Could you check a few things on this model? Use its own coordinates, in mm. A direction names the side the tool comes from. Give positions to 0.01 mm unless a question says otherwise; leave off trailing zeros. Write each loop counter-clockwise with the first axis right and the second up, starting at its lowest first coordinate (ties: lowest second). Pieces come first, ordered by that corner, then holes. Notation, with made-up numbers: M -32.5,82.5 L -25.5,82.5 A27 cw -25.5,102.5 Z; hole C 30,60.5 d5. An arc over 180 degrees is marked long. Answer as CSV lines item,"result". Start each with the question number.
from build123d import *

# Parameters (mm, degrees)
SKETCH_1_W          = 120
SKETCH_1_H          = 155
SKETCH_1_R          = 1.45
SKETCH_1_R_2        = 30.5
SKETCH_1_R_3        = 1.725
SKETCH_1_W_2        = 35
SKETCH_1_H_2        = 28
SKETCH_1_W_3        = 54.975
SKETCH_1_H_3        = 45
SKETCH_1_W_4        = 4.95
SKETCH_1_H_4        = 20
EXTRUDE_1_DEPTH     = 3
FILLET_1_R          = 6
FILLET_2_R          = 10
SKETCH_2_W          = 31.025
SKETCH_2_H          = 25
CUT_EXTRUDE_1_DEPTH = 197.04591299
FILLET_3_R          = 6
FILLET_4_R          = 5
SKETCH_3_R          = 1.5
CUT_EXTRUDE_2_DEPTH = 197.04591299


with BuildPart() as part:
    # 草图1 → 凸台-拉伸1 (new body)
    # profile 1 of 2: a face of its own
    with BuildSketch(Plane.XY):
        with Locations((-60, 77.5)):
            Rectangle(SKETCH_1_W, SKETCH_1_H)
        with Locations((-15, 7.5)):
            Circle(SKETCH_1_R, mode=Mode.SUBTRACT)
        with Locations((-55, 7.5)):
            Circle(SKETCH_1_R, mode=Mode.SUBTRACT)
        with Locations((-15, 147.5)):
            Circle(SKETCH_1_R, mode=Mode.SUBTRACT)
        with Locations((-55, 147.5)):
            Circle(SKETCH_1_R, mode=Mode.SUBTRACT)
        with Locations((-56.5, 92)):
            Circle(SKETCH_1_R_2, mode=Mode.SUBTRACT)
        with Locations((-56.5, 134.5)):
            Circle(SKETCH_1_R_3, mode=Mode.SUBTRACT)
        with Locations((-56.5, 49.5)):
            Circle(SKETCH_1_R_3, mode=Mode.SUBTRACT)
        with Locations((-87.966251763, 123.466251763)):
            Circle(SKETCH_1_R_3, mode=Mode.SUBTRACT)
        with Locations((-87.966251763, 60.533748237)):
            Circle(SKETCH_1_R_3, mode=Mode.SUBTRACT)
        with Locations((-25.033748237, 60.533748237)):
            Circle(SKETCH_1_R_3, mode=Mode.SUBTRACT)
        with Locations((-25.033748237, 123.466251763)):
            Circle(SKETCH_1_R_3, mode=Mode.SUBTRACT)
        with Locations((-12, 92)):
            Circle(SKETCH_1_R_3, mode=Mode.SUBTRACT)
        with Locations((-101, 92)):
            Circle(SKETCH_1_R_3, mode=Mode.SUBTRACT)
        with Locations((-95, 7.5)):
            Circle(SKETCH_1_R, mode=Mode.SUBTRACT)
        with Locations((-95, 147.5)):
            Circle(SKETCH_1_R, mode=Mode.SUBTRACT)
        Polygon((-110, 65), (-110, 15), (-85, 15), (-85, 45), align=None, mode=Mode.SUBTRACT)
        with Locations((-57.5, 29)):
            Rectangle(SKETCH_1_W_2, SKETCH_1_H_2, mode=Mode.SUBTRACT)
        Polygon((-10, 60), (-10, 15), (-30, 15), (-30, 45), align=None, mode=Mode.SUBTRACT)
    # profile 2 of 2: a face of its own
    with BuildSketch(Plane.XY):
        with Locations((27.4875, 105)):
            Rectangle(SKETCH_1_W_3, SKETCH_1_H_3)
        with Locations((41, 102.5)):
            Circle(SKETCH_1_R, mode=Mode.SUBTRACT)
        with Locations((41, 112.5)):
            Circle(SKETCH_1_R, mode=Mode.SUBTRACT)
        with Locations((47.5, 107.5)):
            Rectangle(SKETCH_1_W_4, SKETCH_1_H_4, mode=Mode.SUBTRACT)
    extrude(amount=EXTRUDE_1_DEPTH)

    # 圆角1
    fillet_1_edges = [part.edges().sort_by_distance(p)[0] for p in [
        (-75, 43, 1.5),
        (-75, 15, 1.5),
        (-40, 15, 1.5),
        (-40, 43, 1.5),
        (-110, 65, 1.5),
        (-110, 15, 1.5),
        (-85, 15, 1.5),
        (-85, 45, 1.5),
        (-30, 15, 1.5),
        (-10, 15, 1.5),
        (-10, 60, 1.5),
        (-30, 45, 1.5),
    ]]
    fillet(fillet_1_edges, radius=FILLET_1_R)

    # 圆角2
    fillet_2_edges = [part.edges().sort_by_distance(p)[0] for p in [
        (0, 82.5, 1.5),
        (0, 127.5, 1.5),
    ]]
    fillet(fillet_2_edges, radius=FILLET_2_R)

    # 草图2 → 切除-拉伸1 (cut, through all)
    with BuildSketch(Plane.XY.offset(3)):
        with Locations((17.5125, 105)):
            Rectangle(SKETCH_2_W, SKETCH_2_H)
    extrude(amount=-CUT_EXTRUDE_1_DEPTH, mode=Mode.SUBTRACT)

    # 圆角3
    fillet_3_edges = [part.edges().sort_by_distance(p)[0] for p in [
        (2, 92.5, 1.5),
        (2, 117.5, 1.5),
        (33.025, 117.5, 1.5),
        (33.025, 92.5, 1.5),
    ]]
    fillet(fillet_3_edges, radius=FILLET_3_R)

    # 圆角4
    fillet_4_edges = [part.edges().sort_by_distance(p)[0] for p in [
        (54.975, 82.5, 1.5),
        (0, 0, 1.5),
        (-120, 0, 1.5),
        (-120, 155, 1.5),
        (0, 155, 1.5),
        (54.975, 127.5, 1.5),
    ]]
    fillet(fillet_4_edges, radius=FILLET_4_R)

    # 草图3 → 切除-拉伸2 (cut, through all)
    with BuildSketch(Plane.XY.offset(3)):
        with Locations((45.025, 117.5)):
            Circle(SKETCH_3_R)
        with Locations((49.975, 117.5)):
            Circle(SKETCH_3_R)
        with Locations((45.025, 97.5)):
            Circle(SKETCH_3_R)
        with Locations((49.975, 97.5)):
            Circle(SKETCH_3_R)
    extrude(amount=-CUT_EXTRUDE_2_DEPTH, mode=Mode.SUBTRACT)


solid = part.part
1. Please list where these lines run through material, in increasing order: line 1 (Y direction, x = -56.5, z = 1.2) (3 decimals); line 2 (X direction, y = 59.5, z = 1.2); line 3 (Y direction, x = -104.5, z = 1.1).
2. Imagine slicing it at D-D, the plane y = 141. Please give me the cut outline in (x, z), plus the area to 3 significant figures.
3. Imagine slicing it at B-B, the plane y = 65. Please give me the cut outline in (x, z), plus the area to 3 significant figures.
4. Imagine slicing it at C-C, the plane z = 1.4. State how many separate pieces and enclosed holes the cut face has, plus the area to 3 significant figures.
5. Will these pins go through, and if not, where does the flat tip stop? P1, Ø0.9, axis at y = 26.5, z = 1, coming from the +X side; P2, Ø0.9, axis at x = 21, z = 2, coming from the +Y side; P3, Ø1.5, axis at x = 20.5, z = 1.5, coming from the -Y side.
6. On a 3-axis mill with a long thin cutter (end or side, diameter ignored), from which of +Z, -Z, +X, -X, +Y, -Y can I reach the whole of each face in a straight line? I mean faces 4 (the cylindrical face through (-1, 2, 2)), 5 (the cylindrical face through (-108.289, 16.804, 1.521)). Say none if no direction works.
7. Thinking about a two-plate mould opening in Y: for faces 1 (the cylindrical face through (-119, 153, 2)), 2 (the cylindrical face through (2.85, 79.49, 1.52)), 3 (the cylindrical face through (-80.704, 73.441, 1.479)), which applies, pulls with the +Y half, pulls with the -Y half, needs draft (parallel to the pull), parting line crosses it, or undercut?
8. Imagine slicing it at A-A, the plane x = -37. Please give me the cut outline in (y, z), plus the area to 3 significant figures.
Solutions:
1,line 1,"0 to 15, 43 to 47.775, 51.225 to 61.5, 122.5 to 132.775, 136.225 to 155"
1,line 2,"-120 to -89.35, -86.59 to -26.41, -23.65 to 0"
1,line 3,"0 to 15.02, 58.5 to 155"
2,outline,"M -120,0 L 0,0 L 0,3 L -120,3 Z"
2,area,"360 mm²"
3,outline,"M -120,0 L -70.69,0 L -70.69,3 L -120,3 Z; M -42.31,0 L 0,0 L 0,3 L -42.31,3 Z"
3,area,"275 mm²"
4,separate pieces,"1"
4,enclosed holes,"22"
4,area,"14,600 mm²"
5,P1,"x = 0"
5,P2,"y = 127.5"
5,P3,"y = 82.5"
6,face 4,"+Z, -Z, +X, -Y"
6,face 5,"+Z, -Z"
7,face 1,"pulls with the +Y half"
7,face 2,"pulls with the -Y half"
7,face 3,"undercut"
8,outline,"M 0,0 L 68.55,0 L 68.55,3 L 0,3 Z; M 115.45,0 L 155,0 L 155,3 L 115.45,3 Z"
8,area,"324 mm²"
